Geometry: see drawing. Coordinates: mm, zero at the bounding-box minimum. A direction names the side the tool comes from. Give positions to 0.01 mm unless a question says otherwise; leave off trailing zeros. Order: outer loops, then holes, each group sorted by start corner. A loop starts at its lowest first (then second) coordinate and runs counter-clockwise, first axis right, second up. Notation, with made-up numbers: (82.25, -18) - (139.25, -18) arc R17 cw to (139.25, -6) - close; hole circle Ø8 at (44.5, 0.25). An arc over 180 degrees is marked (long way). One line per item, written item: value.
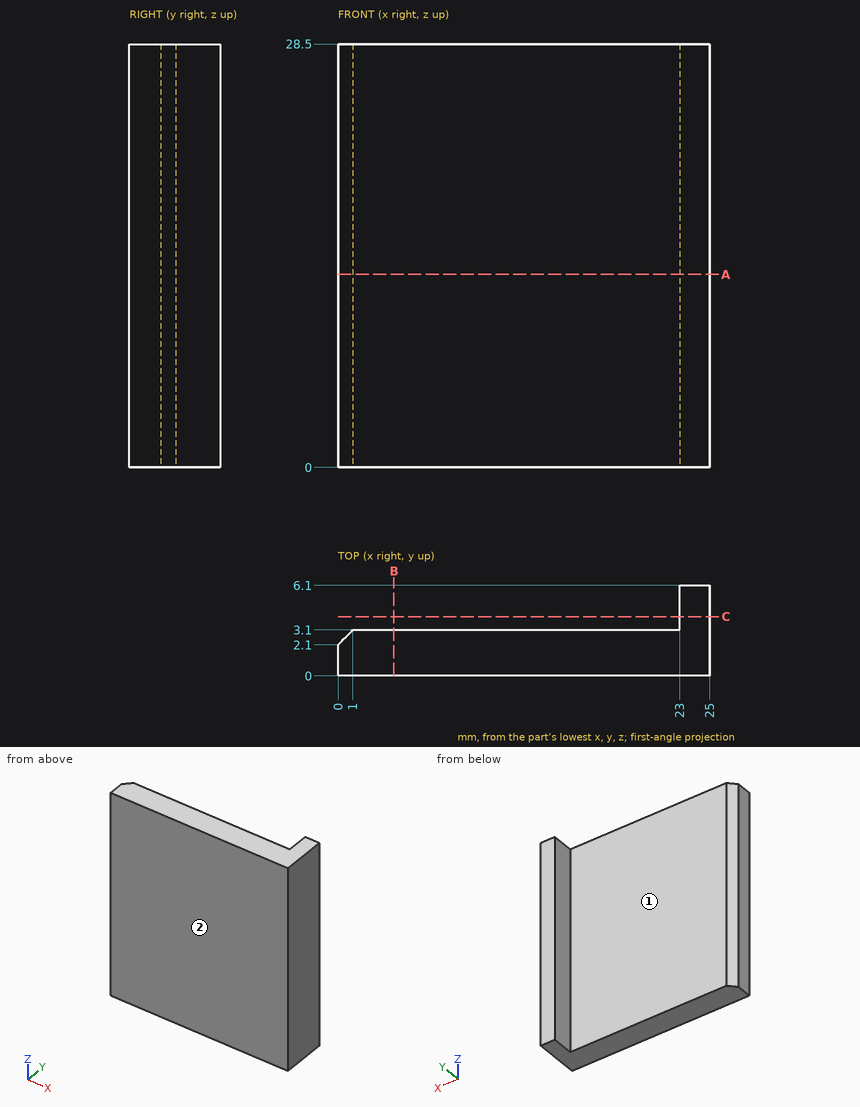
1) First-contact query: pin 1 (5 mm diameter, centred on x = 20, z = 21, fed in from +Y); pin 2 (2.5 mm diameter, centred on y = 5, z = 8, fed in from -X). Flat tips, straight axial feed; report the tip coordinate or a pass-through.
Answers below:
pin 1: y = 3.1
pin 2: x = 23
2) Section B-B, the plane x = 3.75. Return loops of the section in (y, z).
Answers below:
outline: (0, 0) - (3.1, 0) - (3.1, 28.5) - (0, 28.5) - close
3) Set-up query: the marked faces 1 and 2. Return all of +Z, -Z, +X, -X, +Y, -Y with unobstructed straight access to the full face (end or side cutting, diameter ignored); none if empty.
Answers below:
face 1: +Z, -Z, -X, +Y
face 2: +Z, -Z, +X, -X, -Y
4) Section C-C, the plane y = 4. Return loops of the section in (x, z).
Answers below:
outline: (23, 0) - (25, 0) - (25, 28.5) - (23, 28.5) - close
5) Material intervals for line 1 along X through (y, z) = (5, 22); line 2 along Y through (x, z) = (10.25, 6.5), sorted ascending.
Answers below:
line 1: 23 to 25
line 2: 0 to 3.1
6) Section A-A, the plane z = 13. Return loops of the section in (x, y), then the cut area to 3 significant figures.
Answers below:
outline: (0, 0) - (25, 0) - (25, 6.1) - (23, 6.1) - (23, 3.1) - (1, 3.1) - (0, 2.1) - close
area: 83.0 mm^2
